Could you check a few things on this drawing? It's one solid part, dimensions in mm from its lowest x, y, z. Give positions to 0.01 mm unless a question says otherwise; leave off trailing zeros. Order: outer loops, then holes, each group sorted by start corner. A loop starts at its lowest first (then second) coordinate and runs counter-clockwise, first axis right, second up.
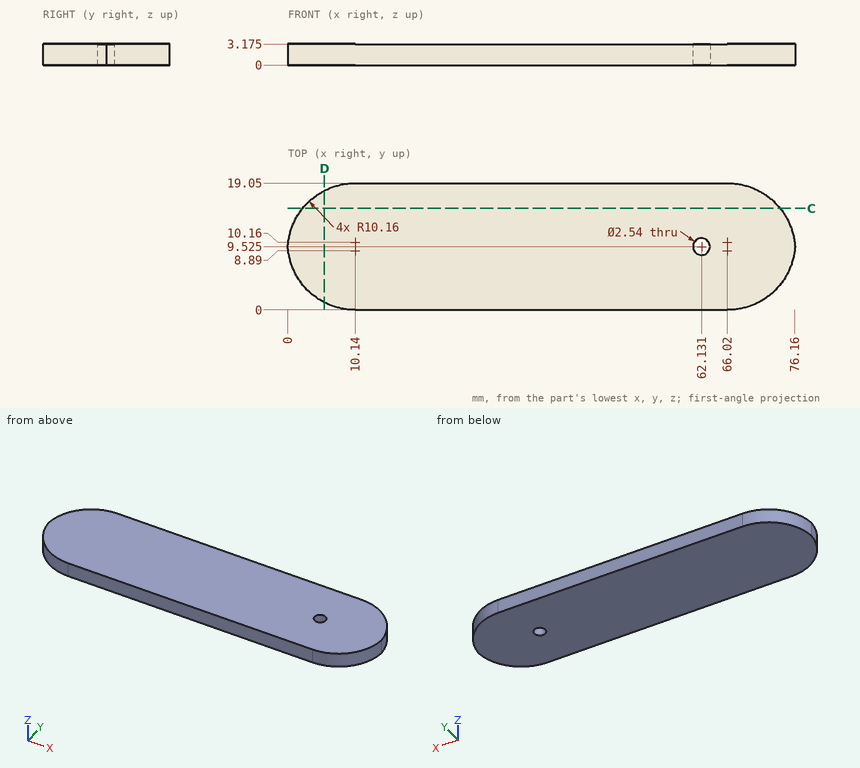
Q1. If we section it at D-D on x = 5.5: List the corners of the cut face in (y, z) for me (1 decimal).
Filled sheet:
outline: (1.1, 0) - (17.9, 0) - (17.9, 3.2) - (1.1, 3.2) - close
Q2. If we section it at C-C on y = 15.25: List the corners of the cut face in (x, z) for me (1 decimal), plus the area to 3 significant figures.
Filled sheet:
outline: (2.2, 0) - (73.9, 0) - (73.9, 3.2) - (2.2, 3.2) - close
area: 228 mm2
Q3. I need wall thicknesses on L1, parallel to X at y = 8.5, z = 1.9 (1 decimal); L2, parallel to X at y = 14.5, z = 0.35; L3, parallel to Y at x = 9, z = 1.75 (1 decimal). Which ranges of each line are inside material? Lowest first, please.
Filled sheet:
L1: x = 0.1 to 61.4, 62.9 to 76
L2: x = 1.67 to 74.49
L3: y = 0.1 to 19
